Input: part model. Units: mm. Frame: model coordinates. Coordinates: 2 decimals unless noted, no trailing zeros. Order: outer loops, then holes, each group sorted by start corner. A loop starts at its lowest first (then second) coordinate and runs counter-clockwise, first axis right, second up. Notation, with made-up numbers: M 12,21 L 41,21 A12 cw 41,34 Z; hole C 56.5,-8.75 d2. An arc over 180 degrees is marked long. One line per item, written item: value.
```python
from build123d import *

# Parameters (mm, degrees)
BOSS_EXTRUDE1_DEPTH = 12


with BuildPart() as part:
    # Sketch1 → Boss-Extrude1 (new body)
    with BuildSketch(Plane.XY):
        with BuildLine():
            Line((511.8067094, 188.903885219), (511.8067094, 142.299329353))
            ThreePointArc((511.8067094, 142.299329353), (511.806507744, 138.903885219), (515.20195099, 138.906348311))
            Line((515.20195099, 138.906348311), (523.8067094, 138.906348311))
            Line((523.8067094, 138.906348311), (523.8067094, 138.319810176))
            Line((523.8067094, 138.319810176), (523.8067094, 88.903885219))
            Line((523.8067094, 88.903885219), (518.8067094, 88.903885219))
            Line((518.8067094, 88.903885219), (515.20195099, 88.903885219))
            ThreePointArc((515.20195099, 88.903885219), (511.806507744, 88.906348311), (511.8067094, 85.510904177))
            Line((511.8067094, 85.510904177), (511.8067094, 42.296866261))
            ThreePointArc((511.8067094, 42.296866261), (511.806507744, 38.901422127), (515.20195099, 38.903885219))
            Line((515.20195099, 38.903885219), (518.8067094, 38.903885219))
            Line((518.8067094, 38.903885219), (523.8067094, 38.903885219))
            Line((523.8067094, 38.903885219), (523.8067094, -11.096114781))
            Line((523.8067094, -11.096114781), (518.8067094, -11.096114781))
            Line((518.8067094, -11.096114781), (515.20195099, -11.096114781))
            ThreePointArc((515.20195099, -11.096114781), (511.806507744, -11.093651689), (511.8067094, -14.489095823))
            Line((511.8067094, -14.489095823), (511.8067094, -57.703133739))
            ThreePointArc((511.8067094, -57.703133739), (511.806507744, -61.098577873), (515.20195099, -61.096114781))
            Line((515.20195099, -61.096114781), (518.8067094, -61.096114781))
            Line((518.8067094, -61.096114781), (523.8067094, -61.096114781))
            Line((523.8067094, -61.096114781), (523.8067094, -111.096114781))
            Line((523.8067094, -111.096114781), (518.8067094, -111.096114781))
            Line((518.8067094, -111.096114781), (515.20195099, -111.096114781))
            ThreePointArc((515.20195099, -111.096114781), (511.806507744, -111.093651689), (511.8067094, -114.489095823))
            Line((511.8067094, -114.489095823), (511.8067094, -161.096114781))
            Line((511.8067094, -161.096114781), (-613.922135209, -161.096114781))
            Line((-613.922135209, -161.096114781), (-613.922135209, -114.489095823))
            ThreePointArc((-613.922135209, -114.489095823), (-613.921933554, -111.093651689), (-617.3173768, -111.096114781))
            Line((-617.3173768, -111.096114781), (-620.922135209, -111.096114781))
            Line((-620.922135209, -111.096114781), (-625.922135209, -111.096114781))
            Line((-625.922135209, -111.096114781), (-625.922135209, -61.096114781))
            Line((-625.922135209, -61.096114781), (-620.922135209, -61.096114781))
            Line((-620.922135209, -61.096114781), (-617.3173768, -61.096114781))
            ThreePointArc((-617.3173768, -61.096114781), (-613.921933554, -61.098577873), (-613.922135209, -57.703133739))
            Line((-613.922135209, -57.703133739), (-613.922135209, -14.489095823))
            ThreePointArc((-613.922135209, -14.489095823), (-613.921933554, -11.093651689), (-617.3173768, -11.096114781))
            Line((-617.3173768, -11.096114781), (-620.922135209, -11.096114781))
            Line((-620.922135209, -11.096114781), (-625.922135209, -11.096114781))
            Line((-625.922135209, -11.096114781), (-625.922135209, 38.903885219))
            Line((-625.922135209, 38.903885219), (-620.922135209, 38.903885219))
            Line((-620.922135209, 38.903885219), (-617.3173768, 38.903885219))
            ThreePointArc((-617.3173768, 38.903885219), (-613.921933554, 38.901422127), (-613.922135209, 42.296866261))
            Line((-613.922135209, 42.296866261), (-613.922135209, 85.510904177))
            ThreePointArc((-613.922135209, 85.510904177), (-613.921933554, 88.906348311), (-617.3173768, 88.903885219))
            Line((-617.3173768, 88.903885219), (-620.922135209, 88.903885219))
            Line((-620.922135209, 88.903885219), (-625.922135209, 88.903885219))
            Line((-625.922135209, 88.903885219), (-625.922135209, 138.319810176))
            Line((-625.922135209, 138.319810176), (-625.922135209, 138.906348311))
            Line((-625.922135209, 138.906348311), (-617.3173768, 138.906348311))
            ThreePointArc((-617.3173768, 138.906348311), (-613.921933554, 138.903885219), (-613.922135209, 142.299329353))
            Line((-613.922135209, 142.299329353), (-613.922135209, 188.903885219))
            Line((-613.922135209, 188.903885219), (511.8067094, 188.903885219))
        make_face()
    extrude(amount=BOSS_EXTRUDE1_DEPTH)


solid = part.part
```
(1) Cut plane A-A on y = 63.5. Output: boundary loops of the cut face in (x, z).
Data:
outline: M -613.92,0 L 511.81,0 L 511.81,12 L -613.92,12 Z
(2) First-contact query: pin 1 (2.5 mm diameter, centred on x = 517.5, z = 4.5, fed in from +Y); pin 2 (10 mm diameter, centred on x = 85.5, y = 50.5, fed in from -Z); pin 3 (4.5 mm diameter, centred on x = 518, z = 5, fed in from -Y); pin 4 (3.5 mm diameter, centred on y = 68.5, z = 6.5, fed in from -X). Flat tips, straight axial feed; report the tip coordinate or a pass-through.
Data:
pin 1: stops at y = 138.91
pin 2: stops at z = 0
pin 3: stops at y = -111.1
pin 4: stops at x = -613.92
(3) Ray query, line 1 (X direction, y = 84, z = 3); line 2 (X direction, y = -14, z = 5.5). Return the intervals inside material, ascending. Write a range as from..to.
Data:
line 1: x = -613.92..511.81
line 2: x = -613.55..511.43
(4) Draft query along Z for faces 1 (the flat face through (-43, 16, 0)), 2 (the flat face through (-43, 16, 12)). Return one class per face: released by +Z, released by -Z, zero draft, split by the parting line, or undercut.
Data:
face 1: released by -Z
face 2: released by +Z
